Part model, mm, in its own coordinate system. A direction names the side the tool comes from. Give positions to 0.01 mm unless a question says otherwise; leave off trailing zeros. Write each loop counter-clockwise with the first axis right and the second up, starting at its lowest first coordinate (ties: lowest second). Pieces come first, ordered by that corner, then holes. Notation, with made-up numbers: M 58,7.5 L 117,7.5 A17 ccw 117,14.5 Z; hole C 81,-35.75 d11. An arc over 180 degrees is marked long. Use CSV: the item, a comma, the result in double quotes. Start each with the question number.
1. Band-saw the part on C-C, the plane x = -29.5. List the corners of the cut face in (y, z), then the cut area to 3 significant figures.
2. 3-axis set-ups, long thin cutter, end or side, ignore diameter. For faces 4 (the face through (0.911, -89, 27)), 5 (the face through (34, -50.8, -17)), 6 (the face through (-0.62, -88.44, 57.18)), 7 (the face through (-99.24, -125.47, -4.06)), 8 (the face through (-99.24, -64.32, -66.85)): which of +Z, -Z, +X, -X, +Y, -Y reach the whole face in a straight line?
3. Drop flat-ended pins along their axis: pin 1 Ø10 at (x, z) = (31.5, 31) entering from -Y; pin 2 Ø22.5 at (x, y) = (-15, -97.5) entering from -Z; pin 3 Ø16 at (y, z) = (-85.5, 35.5) entering from +X. Give the stop position or say it passes through.
4. Drill centre lines: line 1 along X through (y, z) = (-96, 19); line 2 along Y through (x, z) = (-28, -44); line 3 along X through (y, z) = (-114, -19). Where is each one in solid material? Low to high. Write a range as from..to.
5. Band-saw the part on A-A, the plane y = -96.52. List the corners of the cut face in (x, z), then the cut area to 3 significant figures.
6. Mould opens along Z. For faces 1 (the face through (15.388, -25.756, -37.533)), 2 (the face through (-18.3, -125.6, -3.3)), 3 (the face through (-61, -127, 9)) say: pulls with the +Z half, pulls with the -Z half, needs draft (parallel to the pull), parting line crosses it, or undercut.
7. Band-saw the part on B-B, the plane x = -72. List the corners of the cut face in (y, z), then the cut area to 3 significant figures.
8. Band-saw the part on D-D, the plane y = -79. List the corners of the cut face in (x, z), then the cut area to 3 significant figures.
from build123d import *

# Parameters (mm, degrees)
F0_W     = 203.2
F0_H     = 127
F1_DEPTH = 127
F3_DEPTH = 76.2
F4_SIZE2 = 101.6
F4_SIZE  = 76.2
F5_R     = 5.08
F6_R     = 15.24
F7_DEPTH = 50.8
F8_R     = 12.7
F9_DEPTH = 127


with BuildPart() as f1:
    # F0 (on Front) → F1 (new body)
    with BuildSketch(Plane.XZ):
        with Locations((0.9113103151, -4.8755629536)):
            Rectangle(F0_W, F0_H)
    extrude(amount=F1_DEPTH)

    # F2 (on face) → F3 (cut)
    with BuildSketch(Plane.XZ.offset(127)):
        Polygon((102.5113103151, 58.6244370464), (0.9113103151, 58.6244370464), (0.9113103151, -4.8755629536), (-37.1886896849, -4.8755629536), (-37.1886896849, -68.3755629536), (102.5113103151, -68.3755629536), align=None)
    extrude(amount=-F3_DEPTH, mode=Mode.SUBTRACT)

    # F4
    f4_edges = [f1.edges().sort_by_distance(p)[0] for p in [
        (102.51131, -25.4, 58.624437),
    ]]
    f4_side = f1.faces().sort_by_distance((-20.860118, -52.614286, 58.624437))[0]
    chamfer(f4_edges, length=F4_SIZE, length2=F4_SIZE2, reference=f4_side)

    # F5
    f5_edges = [f1.edges().sort_by_distance(p)[0] for p in [
        (0.91131, -88.9, 58.624437),
        (26.31131, -25.4, 58.624437),
        (13.61131, -50.8, 58.624437),
        (-49.88869, -127, 58.624437),
        (0.91131, -127, 26.874437),
        (0.91131, -88.9, -4.875563),
        (-18.13869, -127, -4.875563),
        (-37.18869, -127, -36.625563),
        (32.66131, -50.8, -68.375563),
        (-37.18869, -88.9, -68.375563),
        (-68.93869, -127, -68.375563),
        (-100.68869, -127, -4.875563),
        (-100.68869, -63.5, 58.624437),
        (-37.18869, 0, 58.624437),
        (102.51131, -25.4, -68.375563),
        (-100.68869, 0, -4.875563),
        (-100.68869, -63.5, -68.375563),
        (0.91131, 0, -68.375563),
        (0.91131, -50.8, 26.874437),
        (-37.18869, -50.8, -36.625563),
        (-37.18869, -88.9, -4.875563),
        (-18.13869, -50.8, -4.875563),
    ]]
    fillet(f5_edges, radius=F5_R)

    # F6 (on face) → F7 (cut, through all)
    with BuildSketch(Plane.XZ.offset(50.8)):
        with Locations((18.6913103151, -22.6555629536)):
            Circle(F6_R)
    extrude(amount=-F7_DEPTH, mode=Mode.SUBTRACT)

    # F8 (on face) → F9 (cut, through all)
    with BuildSketch(Plane.XY.offset(58.6244370464)):
        with Locations((-80.3686896849, -96.52)):
            Circle(F8_R)
    extrude(amount=-F9_DEPTH, mode=Mode.SUBTRACT)


solid = f1.part
Output:
1,outline,"M -127,0.2 A5.08 ccw -121.92,-4.88 L -55.88,-4.88 A5.08 cw -50.8,-9.96 L -50.8,-63.3 A5.08 ccw -45.72,-68.38 L -5.08,-68.38 A5.08 ccw 0,-63.3 L 0,53.54 A5.08 ccw -5.08,58.62 L -121.92,58.62 A5.08 ccw -127,53.54 Z"
1,area,"11,300 mm²"
2,face 4,"+Z, -Z, +X, -Y"
2,face 5,"-Z, +X, -Y"
2,face 6,"+Z, +X, -Y"
2,face 7,"+Z, -Z, -X, -Y"
2,face 8,"-Z, -X, +Y, -Y"
3,pin 1,"stops at y = -50.8"
3,pin 2,"stops at z = -4.88"
3,pin 3,"stops at x = 0.91"
4,line 1,"x = -100.69..-93.06, -67.68..0.91"
4,line 2,"y = -50.8..0"
4,line 3,"x = -100.69..-37.19"
5,outline,"M -100.69,-63.3 A5.08 ccw -95.61,-68.38 L -93.07,-68.38 L -93.07,58.62 L -95.61,58.62 A5.08 ccw -100.69,53.54 Z; M -67.67,-68.38 L -42.27,-68.38 A5.08 ccw -37.19,-63.3 L -37.19,-9.96 A5.08 cw -32.11,-4.88 L -4.17,-4.88 A5.08 ccw 0.91,0.2 L 0.91,53.54 A5.08 ccw -4.17,58.62 L -67.67,58.62 Z"
5,area,"7,240 mm²"
6,face 1,"undercut"
6,face 2,"pulls with the -Z half"
6,face 3,"needs draft"
7,outline,"M -127,-63.3 A5.08 ccw -121.92,-68.38 L -106.07,-68.38 L -106.07,58.62 L -121.92,58.62 A5.08 ccw -127,53.54 Z; M -86.97,-68.38 L -5.08,-68.38 A5.08 ccw 0,-63.3 L 0,53.54 A5.08 ccw -5.08,58.62 L -86.97,58.62 Z"
7,area,"13,700 mm²"
8,outline,"M -100.69,-63.3 A5.08 ccw -95.61,-68.38 L -42.27,-68.38 A5.08 ccw -37.19,-63.3 L -37.19,-9.96 A5.08 cw -32.11,-4.88 L -4.17,-4.88 A5.08 ccw 0.91,0.2 L 0.91,53.54 A5.08 ccw -4.17,58.62 L -95.61,58.62 A5.08 ccw -100.69,53.54 Z"
8,area,"10,500 mm²"
